```python
from build123d import *

# Parameters (mm, degrees)
SKETCH1_W           = 42
SKETCH1_H           = 30
SKETCH1_W_2         = 20
SKETCH1_H_2         = 3
BOSS_EXTRUDE1_DEPTH = 3
SKETCH2_R           = 3.5
SKETCH2_R_2         = 1.525
CUT_EXTRUDE1_DEPTH  = 4


with BuildPart() as part:
    # Sketch1 → Boss-Extrude1 (new body)
    with BuildSketch(Plane.XY):
        Rectangle(SKETCH1_W, SKETCH1_H)
        with Locations((0, 16.5)):
            Rectangle(SKETCH1_W_2, SKETCH1_H_2)
        with Locations((0, -16.5)):
            Rectangle(SKETCH1_W_2, SKETCH1_H_2)
    extrude(amount=BOSS_EXTRUDE1_DEPTH)

    # Sketch2 → Cut-Extrude1 (cut, through all)
    with BuildSketch(Plane.XY.offset(3)):
        with Locations((8.175, 0)):
            Circle(SKETCH2_R)
        with Locations((16.425, 0)):
            Circle(SKETCH2_R_2)
        with Locations((-0.075, 0)):
            Circle(SKETCH2_R_2)
    extrude(amount=-CUT_EXTRUDE1_DEPTH, mode=Mode.SUBTRACT)


solid = part.part
```
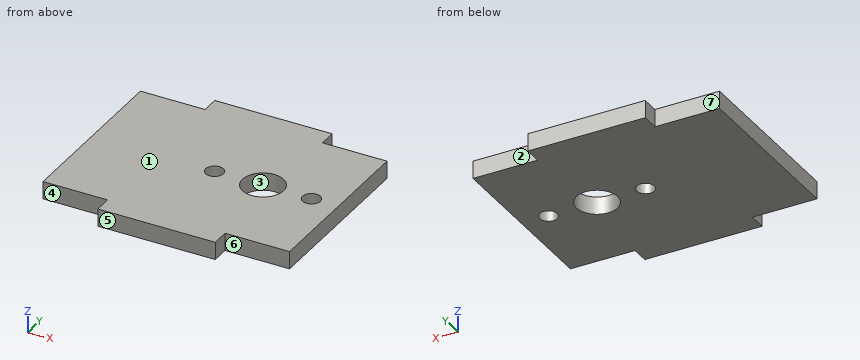
Here's how the part is built. I have some questions about the finished solid (model axes, mm). Face numbers are marked on the shaded views. A direction names the side the tool comes from. Round coordinates to 2 decimals unless told otherwise and drop trailing zeros. Order: outer loops, then holes, each group sorted by start corner. A loop starts at its lowest first (then second) coordinate and runs counter-clockwise, first axis right, second up. Notation, with made-up numbers: M 30,-32.5 L 39,-32.5 A23 ccw 39,3.5 Z; hole C -14,41 d3. An arc over 180 degrees is marked long. Answer in a Markdown table with one row per item.
Item 1: Imagine slicing it at D-D, the plane x = 13. Write out the boundary of the cut face in (y, z).
A:
| item | result |
|---|---|
| outline | M -15,0 L 15,0 L 15,3 L -15,3 Z |
Item 2: I'm going to push flat-ended pins straight in: pin 1 (1 mm diameter, centred on x = -15, z = 1, fed in from +Y); pin 2 (5.5 mm diameter, centred on x = 8.175, y = 0, fed in from +Z); pin 3 (1.5 mm diameter, centred on x = 11.5, z = 0.5, fed in from -Y). Where does each tip first touch, or does it pass through?
A:
| item | result |
|---|---|
| pin 1 | stops at y = 15 |
| pin 2 | passes through |
| pin 3 | stops at y = -15 |
Item 3: If I drill on L1, parallel to Y at x = 19, z = 1.45; L2, parallel to Y at x = 5, z = 0.3; L3, parallel to Y at x = 16, z = 2.15, over which ranges is the centre line in solid material (lowest first)? Write a range as from..to.
A:
| item | result |
|---|---|
| L1 | y = -15..15 |
| L2 | y = -18..-1.47, 1.47..18 |
| L3 | y = -15..-1.46, 1.46..15 |
Item 4: Imagine slicing it at B-B, the plane z = 1.3. Write out the boundary of the cut face in (x, y) (3 decimals).
A:
| item | result |
|---|---|
| outline | M -21,-15 L -10,-15 L -10,-18 L 10,-18 L 10,-15 L 21,-15 L 21,15 L 10,15 L 10,18 L -10,18 L -10,15 L -21,15 Z; hole C -0.075,0 d3.05; hole C 8.175,0 d7; hole C 16.425,0 d3.05 |
Item 5: Imagine slicing it at C-C, the plane x = 0. Write out the boundary of the cut face in (y, z).
A:
| item | result |
|---|---|
| outline | M -18,0 L -1.52,0 L -1.52,3 L -18,3 Z; M 1.52,0 L 18,0 L 18,3 L 1.52,3 Z |
Item 6: Thinking about a two-plate mould opening in Y: for the marked faces 1, 2, 3 and 4, which applies, +Y half, -Y half, draft (parallel to the pull), parting line (faces both ways), or undercut?
A:
| item | result |
|---|---|
| face 1 | draft |
| face 2 | +Y half |
| face 3 | undercut |
| face 4 | -Y half |
Item 7: For the marked faces 5, 6 and 7, which set-ups out of +Z, -Z, +X, -X, +Y, -Y let a thin tool reach every point of the face, with its end or its side?
A:
| item | result |
|---|---|
| face 5 | +Z, -Z, +X, -X, -Y |
| face 6 | +Z, -Z, +X, -Y |
| face 7 | +Z, -Z, -X, +Y |
Item 8: Imagine slicing it at A-A, the plane y = 0. Write out the boundary of the cut face in (x, z) (3 decimals), and give its area (3 significant figures).
A:
| item | result |
|---|---|
| outline | M -21,0 L -1.6,0 L -1.6,3 L -21,3 Z; M 1.45,0 L 4.675,0 L 4.675,3 L 1.45,3 Z; M 11.675,0 L 14.9,0 L 14.9,3 L 11.675,3 Z; M 17.95,0 L 21,0 L 21,3 L 17.95,3 Z |
| area | 86.7 mm2 |
